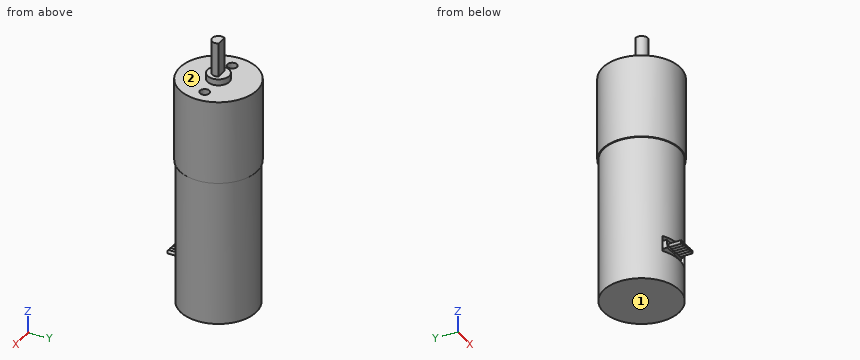
```python
from build123d import *

# Parameters (mm, degrees)
SKETCH1_R           = 12.2
BOSS_EXTRUDE1_DEPTH = 47
SKETCH2_R           = 12.5
BOSS_EXTRUDE2_DEPTH = 27
SKETCH3_R           = 3.5
BOSS_EXTRUDE3_DEPTH = 2
BOSS_EXTRUDE4_DEPTH = 11
SKETCH6_W           = 13
SKETCH6_H           = 5
CUT_EXTRUDE1_DEPTH  = 15
SKETCH7_W           = 8
SKETCH7_H           = 3
BOSS_EXTRUDE6_DEPTH = 2.5
SKETCH8_R           = 0.5
BOSS_EXTRUDE7_DEPTH = 4
DRAFT1_ANGLE        = 5
SKETCH9_R           = 1.55
CUT_EXTRUDE2_DEPTH  = 4


with BuildPart() as part:
    # Sketch1 → Boss-Extrude1 (new body)
    with BuildSketch(Plane.XY):
        Circle(SKETCH1_R)
    extrude(amount=BOSS_EXTRUDE1_DEPTH)

    # Sketch2 → Boss-Extrude2 (add)
    with BuildSketch(Plane.XY.offset(47)):
        Circle(SKETCH2_R)
    extrude(amount=BOSS_EXTRUDE2_DEPTH)

    # Sketch3 → Boss-Extrude3 (add)
    with BuildSketch(Plane.XY.offset(74)):
        Circle(SKETCH3_R)
    extrude(amount=BOSS_EXTRUDE3_DEPTH)

    # Sketch4 → Boss-Extrude4 (add)
    with BuildSketch(Plane.XY.offset(76)):
        with BuildLine():
            Line((-1.732050808, 1), (1.732050808, 1))
            ThreePointArc((1.732050808, 1), (0, -2), (-1.732050808, 1))
        make_face()
    extrude(amount=BOSS_EXTRUDE4_DEPTH)

    # Sketch6 → Cut-Extrude1 (cut)
    with BuildSketch(Plane(origin=(0, 0, 0), x_dir=(1, 0, 0), z_dir=(0, 1, 0))):
        with Locations((0, -12.5)):
            Rectangle(SKETCH6_W, SKETCH6_H)
    extrude(amount=-CUT_EXTRUDE1_DEPTH, mode=Mode.SUBTRACT)

    # Sketch7 → Boss-Extrude6 (add)
    with BuildSketch(Plane(origin=(0, 0, 15), x_dir=(-1, 0, 0), z_dir=(0, 0, -1))):
        with Locations((-0.091140641, -9)):
            Rectangle(SKETCH7_W, SKETCH7_H)
    extrude(amount=BOSS_EXTRUDE6_DEPTH)

    # Sketch8 → Boss-Extrude7 (add)
    with BuildSketch(Plane.XZ.offset(10.5)):
        with Locations((-2.863289538, 13.75)):
            Circle(SKETCH8_R)
        with Locations((-1.663289538, 13.75)):
            Circle(SKETCH8_R)
        with Locations((-0.463289538, 13.75)):
            Circle(SKETCH8_R)
        with Locations((0.736710462, 13.75)):
            Circle(SKETCH8_R)
        with Locations((1.936710462, 13.75)):
            Circle(SKETCH8_R)
        with Locations((3.136710462, 13.75)):
            Circle(SKETCH8_R)
    extrude(amount=BOSS_EXTRUDE7_DEPTH)

    # Draft1
    draft1_faces = [part.faces().sort_by_distance(p)[0] for p in [
        (4.091140641, -9, 13.75),
        (-3.908859359, -9, 13.75),
    ]]
    draft(draft1_faces, Plane(origin=(0, 0, 12.5), x_dir=(-1, 0, 0), z_dir=(0, 0, -1)), DRAFT1_ANGLE)

    # Sketch9 → Cut-Extrude2 (cut)
    with BuildSketch(Plane.XY.offset(74)):
        with Locations((-8, 0)):
            Circle(SKETCH9_R)
        with Locations((8, 0)):
            Circle(SKETCH9_R)
    extrude(amount=-CUT_EXTRUDE2_DEPTH, mode=Mode.SUBTRACT)


solid = part.part
```
For this review, take the finished solid that the model builds, in its own axes (mm). Face numbers are marked on the shaded views. A direction names the side the tool comes from. Coordinates: 2 decimals unless noted, no trailing zeros. Write each loop counter-clockwise with the first axis right and the second up, starting at its lowest first coordinate (ties: lowest second). Pieces come first, ordered by that corner, then holes. Notation, with made-up numbers: (-7.5, 29.5) -> (6.5, 29.5) arc R37 ccw to (6.5, 65.5) -> close; hole circle Ø8 at (14, -3). An arc over 180 degrees is marked (long way). Put each result on its own line as item: value.
Q1. Take a section at A-A, the plane z = 72.5. State the section outline as (x, y) points, then the cut area to 3 significant figures.
From the geometry:
outline: circle Ø25 at (0, 0); hole circle Ø3.1 at (-8, 0); hole circle Ø3.1 at (8, 0)
area: 476 mm2
Q2. Take a section at B-B, the plane x = -8.5. State the section outline as (y, z) points, then the cut area to 3 significant figures.
From the geometry:
outline: (-9.17, 47) -> (-8.75, 47) -> (-8.75, 0) -> (8.75, 0) -> (8.75, 47) -> (9.17, 47) -> (9.17, 74) -> (1.47, 74) -> (1.47, 70) -> (-1.47, 70) -> (-1.47, 74) -> (-9.17, 74) -> close
area: 1,310 mm2
Q3. Wall thickness on L1, parallel to Z at x = 0, y = -0.5; L2, parallel to Z at x = -7.75, y = -0.5; L3, parallel to Z at x = 0, y = 7.5: over which ranges is each line inside the solid? List them lowest first.
From the geometry:
L1: z = 0 to 10, 15 to 87
L2: z = 0 to 70
L3: z = 0 to 74
Q4. Clearance check with flat-ended pins moving along their axes: pin 1 Ø1.6 at (x, y) = (7.5, 0.5) entering from +Z; pin 2 Ø1.5 at (y, z) = (-3, 13.5) entering from -X; pin 3 Ø2 at (x, y) = (4.5, 1) entering from +Z. State where each tip first meets the part, or that it passes through.
From the geometry:
pin 1: stops at z = 70
pin 2: stops at x = -11.99
pin 3: stops at z = 74
Q5. Tool access review of the marked faces 1 and 2: name each direction out of +Z, -Z, +X, -X, +Y, -Y from which nothing blocks a thin tool from reaching the whole face with its end or side.
From the geometry:
face 1: -Z, +X, -X, +Y, -Y
face 2: +Z
Q6. Take a section at C-C, the plane z = 35. State the section outline as (x, y) points.
From the geometry:
outline: circle Ø24.4 at (0, 0)
Q7. Take a section at D-D, the plane x = 10.5. State the section outline as (y, z) points.
From the geometry:
outline: (-6.78, 47) -> (-6.21, 47) -> (-6.21, 0) -> (6.21, 0) -> (6.21, 47) -> (6.78, 47) -> (6.78, 74) -> (-6.78, 74) -> close
